```python
from build123d import *

# Parameters (mm, degrees)
SKETCH_R     = 0.15
PAD_DEPTH    = 1.5
SKETCH001_R  = 0.15
SKETCH002_R  = 1.5875
SKETCH003_R  = 1.5875
PAD001_DEPTH = 33


with BuildPart() as pad:
    # Sketch → Pad (new body)
    with BuildSketch(Plane.XY):
        Circle(SKETCH_R)
    extrude(amount=PAD_DEPTH)


with BuildPart() as pad001:
    # Sketch001 → Loft section 0
    with BuildSketch(Plane.XY.offset(1.5)):
        Circle(SKETCH001_R)
    # Sketch002 → Loft section 1
    with BuildSketch(Plane.XY.offset(5)):
        Circle(SKETCH002_R)
    loft()

    # Fusion: union Pad
    add(pad.part)

    # Sketch003 → Pad001 (new body)
    with BuildSketch(Plane.XY.offset(5)):
        Circle(SKETCH003_R)
    extrude(amount=PAD001_DEPTH)


solid = pad001.part
```
The model under review builds one solid part; all positions refer to its coordinate system, in mm. Give positions to 0.01 mm unless a question says otherwise; leave off trailing zeros. Write each loop counter-clockwise with the first axis right and the second up, starting at its lowest first coordinate (ties: lowest second). Pieces come first, ordered by that corner, then holes. Notation, with made-up numbers: M 66.25,-19.75 L 106.25,-19.75 A17 ccw 106.25,-1.75 Z; hole C 40.5,-36 d8. An arc over 180 degrees is marked long. Write item = value, one per line. Start each with the question number.
Q1. We need section B-B (z = 3). State the section outline as (x, y) points, plus the area to 3 significant figures.
Q2. For line 1 (Y direction, x = 0.15, z = 30); line 2 (X direction, y = 0.9, z = 21); line 3 (Y direction, x = 1.05, z = 18.5), list the stretches that pass through material, from the lowest coordinate up.
Q3. We need section A-A (z = 14). State the section outline as (x, y) points (1 decimal).
Result set:
q1.outline = C 0,0 d1.53
q1.area = 1.84 mm2
q2.line_1 = -1.58 to 1.58
q2.line_2 = -1.31 to 1.31
q2.line_3 = -1.19 to 1.19
q3.outline = C 0,0 d3.2
